Could you check a few things on this model? Use its own coordinates, in mm. Face numbers are marked on the shaded views. A direction names the side the tool comes from. Give positions to 0.01 mm unless a question says otherwise; leave off trailing zeros. Order: outer loops, then holes, each group sorted by start corner. A loop starts at its lowest first (then second) coordinate and runs counter-clockwise, first axis right, second up.
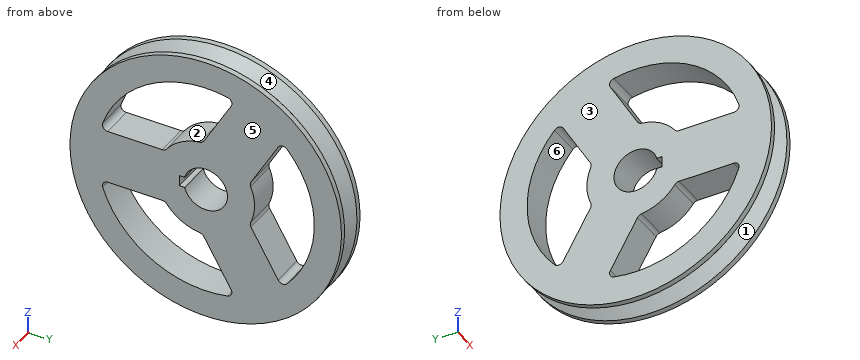
from build123d import *

# Parameters (mm, degrees)
SKETCH1_W           = 30
SKETCH1_H           = 25
BOSS_EXTRUDE1_DEPTH = 15
CUT_EXTRUDE1_DEPTH  = 180.30421077


with BuildPart() as part:
    # Sketch1 → Revolve1 (revolve)
    with BuildSketch(Plane(origin=(0, 0, 0), x_dir=(1, 0, 0), z_dir=(0, 1, 0)), mode=Mode.PRIVATE) as revolve1_sk:
        Polygon((-15, 125), (-15, 100), (15, 100), (15, 125), (10, 125), (0, 115), (-10, 125), align=None)
        with Locations((0, 32.5)):
            Rectangle(SKETCH1_W, SKETCH1_H)
    revolve(revolve1_sk.sketch.rotate(Axis((0, 0, 0), (1, 0, 0)), 180), axis=Axis((0, 0, 0), (1, 0, 0)))

    # Sketch2 → Boss-Extrude1 (add, symmetric)
    with BuildSketch(Plane(origin=(0, 0, 0), x_dir=(0, 0, -1), z_dir=(1, 0, 0))):
        with BuildLine():
            Line((25, -90.138781887), (25, -40))
            ThreePointArc((25, -40), (25.527864045, -37.763932023), (27, -36))
            ThreePointArc((27, -36), (0, -45), (-27, -36))
            ThreePointArc((-27, -36), (-25.527864045, -37.763932023), (-25, -40))
            Line((-25, -40), (-25, -90.138781887))
            ThreePointArc((-25, -90.138781887), (-27.075511741, -94.194317415), (-31.578947368, -94.882928302))
            ThreePointArc((-31.578947368, -94.882928302), (0, -100), (31.578947368, -94.882928302))
            ThreePointArc((31.578947368, -94.882928302), (27.075511741, -94.194317415), (25, -90.138781887))
        make_face()
        with BuildLine():
            ThreePointArc((17.676914536, 41.382685902), (38.97114317, 22.5), (44.676914536, -5.382685902))
            ThreePointArc((44.676914536, -5.382685902), (45.468456501, -3.225812756), (47.141016151, -1.650635095))
            Line((47.141016151, -1.650635095), (90.56247498, 23.418755849))
            ThreePointArc((90.56247498, 23.418755849), (95.112427644, 23.64907772), (97.960499979, 20.093293505))
            ThreePointArc((97.960499979, 20.093293505), (86.602540378, 50), (66.381552611, 74.789634797))
            ThreePointArc((66.381552611, 74.789634797), (68.036915903, 70.545239695), (65.56247498, 66.720026038))
            Line((65.56247498, 66.720026038), (22.141016151, 41.650635095))
            ThreePointArc((22.141016151, 41.650635095), (19.940592456, 40.989744779), (17.676914536, 41.382685902))
        make_face()
        with BuildLine():
            ThreePointArc((-47.141016151, -1.650635095), (-45.468456501, -3.225812756), (-44.676914536, -5.382685902))
            ThreePointArc((-44.676914536, -5.382685902), (-38.97114317, 22.5), (-17.676914536, 41.382685902))
            ThreePointArc((-17.676914536, 41.382685902), (-19.940592456, 40.989744779), (-22.141016151, 41.650635095))
            Line((-22.141016151, 41.650635095), (-65.56247498, 66.720026038))
            ThreePointArc((-65.56247498, 66.720026038), (-68.036915903, 70.545239695), (-66.381552611, 74.789634797))
            ThreePointArc((-66.381552611, 74.789634797), (-86.602540378, 50), (-97.960499979, 20.093293505))
            ThreePointArc((-97.960499979, 20.093293505), (-95.112427644, 23.64907772), (-90.56247498, 23.418755849))
            Line((-90.56247498, 23.418755849), (-47.141016151, -1.650635095))
        make_face()
    extrude(amount=BOSS_EXTRUDE1_DEPTH, both=True)

    # Sketch4 → Cut-Extrude1 (cut, through all)
    with BuildSketch(Plane.ZY.offset(15)):
        with BuildLine():
            Line((5, -24.364916731), (5, -19.364916731))
            ThreePointArc((5, -19.364916731), (0, -20), (-5, -19.364916731))
            Line((-5, -19.364916731), (-5, -24.364916731))
            Line((-5, -24.364916731), (5, -24.364916731))
        make_face()
    extrude(amount=-CUT_EXTRUDE1_DEPTH, mode=Mode.SUBTRACT)


solid = part.part
Item 1: Imagine slicing it at A-A on x = 6. Give the number of separate pieces and of enclosed holes in the cut face, then the cut area to 3 significant figures.
Findings:
separate pieces: 1
enclosed holes: 4
area: 28,200 mm2
Item 2: For the marked faces 4, 5 and 6, which set-ups out of +Z, -Z, +X, -X, +Y, -Y let a thin tool reach every point of the face, with its end or its side?
Findings:
face 4: none
face 5: +Z, -Z, +X, +Y, -Y
face 6: +X, -X
Item 3: We'd pull the mould along Y, two halves only. Please class the marked faces 1, 2 and 3: +Y half, -Y half, draft (parallel to the pull), parting line (faces both ways), or undercut.
Findings:
face 1: parting line
face 2: undercut
face 3: draft
Item 4: Imagine slicing it at B-B on z = 0. List the corners of the cut face in (x, y) for me.
Findings:
outline: (-15, -125) - (-10, -125) - (0, -115) - (10, -125) - (15, -125) - (15, -24.36) - (-15, -24.36) - close; (-15, 20) - (15, 20) - (15, 45) - (-15, 45) - close; (-15, 100) - (15, 100) - (15, 125) - (10, 125) - (0, 115) - (-10, 125) - (-15, 125) - close
Item 5: For pin 1 (8 mm diameter, centred on x = 0.5, z = -2, fed in from +Y); pin 2 (3 mm diameter, centred on x = 5, z = -66.5, fed in from -Y); pin 3 (6 mm diameter, centred on x = -3, y = -96.5, fed in from -Z), each with a flat end and sliding along its axis, tell me the tip position at first contact or that it passes through.
Findings:
pin 1: stops at y = 119.48
pin 2: stops at y = -101.93
pin 3: stops at z = -74.35
Item 6: Please list where these lines run through material, in increasing order: line 1 along Z through (x, y) = (-0.5, -15.5); line 2 along Z through (x, y) = (13.5, -45); line 3 along Z through (x, y) = (-1.25, -76).
Findings:
line 1: z = -114.46 to -98.79, -42.25 to -12.64, 12.64 to 42.25, 98.79 to 114.46
line 2: z = -116.62 to -89.3, -25 to 25, 89.3 to 116.62
line 3: z = -87.97 to -64.99, -25 to 25, 64.99 to 87.97
